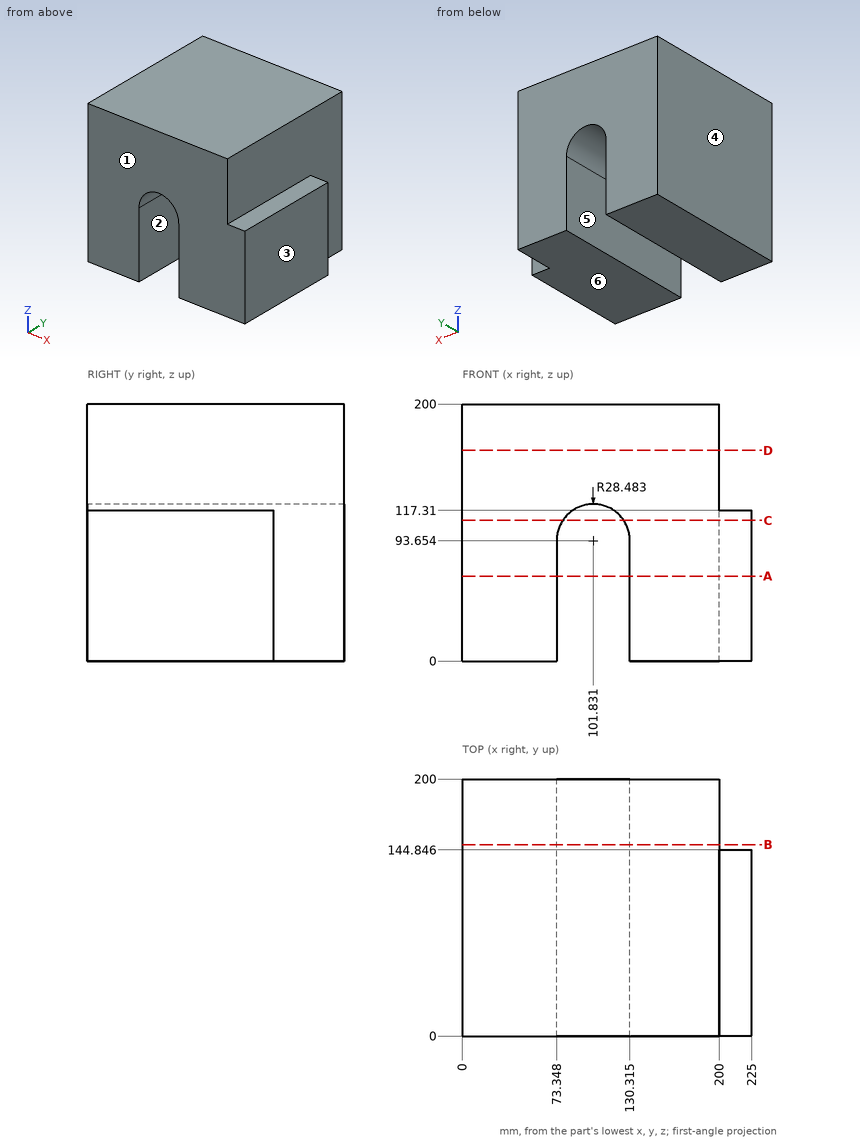
Here's the drawing with two shaded views (mm, measured from the low corner). I have some questions. A direction names the side the tool comes from. Give positions to 0.01 mm unless a question says otherwise; leave off trailing zeros. Order: outer loops, then holes, each group sorted by start corner. A loop starts at its lowest first (then second) coordinate and runs counter-clockwise, first axis right, second up. Notation, with made-up numbers: M -37,50.5 L -22,50.5 A8 cw -22,62.5 Z; hole C -15.5,78 d10. An arc over 180 degrees is marked long. Answer as a JSON object with one key per item and string values. Group by question number.
1) Suppose I cut it at A-A, the plane z = 66. Write out the boundary of the cut face in (x, y) (1 decimal).
2) We'd pull the mould along X, two halves only. Please class the marked faces 3, 4, 5 and 6: pulls with the +X half, pulls with the -X half, needs draft (parallel to the pull), parting line crosses it, or undercut.
3) Suppose I cut it at C-C, the plane z = 109.5. Write out the boundary of the cut face in (x, y).
4) I'm going to push flat-ended pins straight in: pin 1 Ø1 at (y, z) = (158.5, 69) entering from -X; pin 2 Ø1.5 at (y, z) = (90.5, 128) entering from +X. Where does each tip first touch, or does it pass through?
5) Suppose I cut it at D-D, the plane z = 164. Write out the boundary of the cut face in (x, y).
6) Please list where these lines run through material, in increasing order: L1, parallel to X at y = 62, z = 51 (1 decimal); L2, parallel to X at y = 168, z = 88 (1 decimal); L3, parallel to X at y = 101.5, z = 180.5. Write a range as [from, to].
7) Suppose I cut it at B-B, the plane y = 149. Write out the boundary of the cut face in (x, z) (1 decimal).
8) On a 3-axis mill with a long thin cutter (end or side, diameter ignored), from which of +Z, -Z, +X, -X, +Y, -Y can I reach the whole of each face in a straight line? I mean the marked faces 1 and 2. Say none if no direction works.
Results found:
{
 "1": {"outline": "M 0,0 L 73.3,0 L 73.3,200 L 0,200 Z; M 130.3,0 L 225,0 L 225,144.8 L 200,144.8 L 200,200 L 130.3,200 Z"},
 "2": {"face 3": "pulls with the +X half", "face 4": "pulls with the -X half", "face 5": "undercut", "face 6": "needs draft"},
 "3": {"outline": "M 0,0 L 78.16,0 L 78.16,200 L 0,200 Z; M 125.5,0 L 225,0 L 225,144.85 L 200,144.85 L 200,200 L 125.5,200 Z"},
 "4": {"pin 1": "x = 0", "pin 2": "x = 200"},
 "5": {"outline": "M 0,0 L 200,0 L 200,200 L 0,200 Z"},
 "6": {"L1": "[0, 73.3], [130.3, 225]", "L2": "[0, 73.3], [130.3, 200]", "L3": "[0, 200]"},
 "7": {"outline": "M 0,0 L 73.3,0 L 73.3,93.7 A28.5 cw 130.3,93.7 L 130.3,0 L 200,0 L 200,200 L 0,200 Z"},
 "8": {"face 1": "+Z, -Z, +X, -X, -Y", "face 2": "-Z, +Y, -Y"}
}
